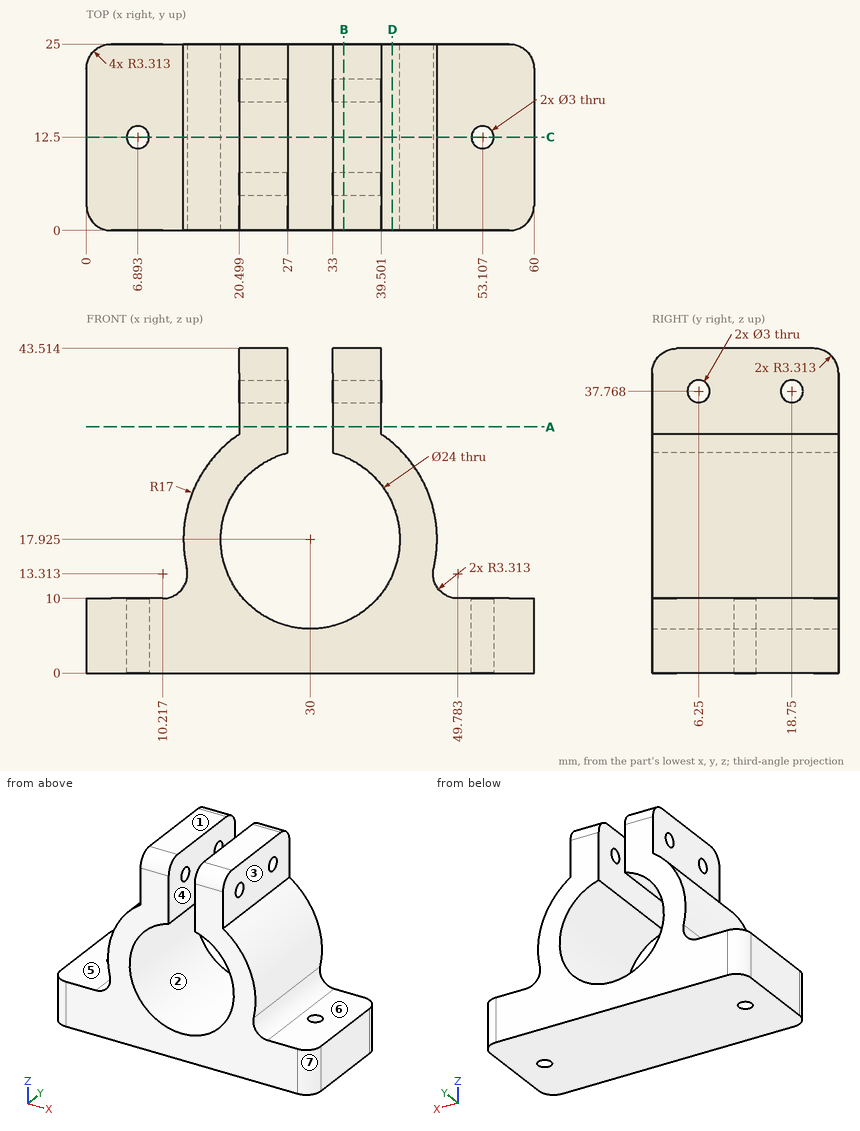
Input: dimensioned drawing with shaded views. Units: mm. Origin: part minimum x, y, z. A direction names the side the tool comes from. Round coordinates to 2 decimals unless told otherwise and drop trailing zeros. Write each loop counter-clockwise with the first axis right and the second up, starting at its lowest first coordinate (ties: lowest second). Pieces come first, ordered by that corner, then holes. Notation, with made-up numbers: (82, 52.5) -> (131, 52.5) arc R17 cw to (131, 83.5) -> close; hole circle Ø7 at (69.25, 12). An arc over 180 degrees is marked (long way). Use CSV: the item, a comma, the result in double quotes. Start each with the question number.
Q1. Reachability of the marked faces 4, 5, 6 and 7 from +Z, -Z, +X, -X, +Y, -Y: full face, straight path, thin tool, end or side. Return the list, or none.
Q2. Section B-B (x = 34.5). Return loops of the section in (y, z).
Q3. Section A-A (z = 33). Return loops of the section in (x, y).
Q4. Section C-C (y = 12.5). Return loops of the section in (x, z) (1 decimal), plus the area to 3 significant figures.
Q5. Pull-direction query (Z, two-part tool) for the marked faces 1, 2 and 3; classes: pulls with the +Z half, pulls with the -Z half, needs draft (parallel to the pull), parting line crosses it, or undercut.
Q6. Section D-D (x = 41). Return loops of the section in (y, z), plus the area to 3 significant figures.
Q7. First-contact query: pin 1 Ø4 at (y, z) = (12, 38) entering from -X; pin 2 Ø5 at (y, z) = (18.75, 37.77) entering from +X; pin 3 Ø3.5 at (x, y) = (53.11, 12.5) entering from +Z. Flat tips, straight axial feed; report the tip coordinate or a pass-through.
Q8. Line query: L1, parallel to X at y = 18.75, z = 34; L2, parallel to Z at x = 36.75, y = 18.75 (1 decimal); L3, parallel to Z at x = 24.5, y = 6.25 (1 decimal). Output: solid intervals per line, ascending.
Result sheet:
1,face 4,"+Z, +Y, -Y"
1,face 5,"+Z, -X, +Y, -Y"
1,face 6,"+Z, +X, +Y, -Y"
1,face 7,"+Z, -Z, +X, -Y"
2,outline,"(0, 0) -> (25, 0) -> (25, 6.8) -> (0, 6.8) -> close; (0, 29.05) -> (25, 29.05) -> (25, 40.2) arc R3.31 ccw to (21.69, 43.51) -> (3.31, 43.51) arc R3.31 ccw to (0, 40.2) -> close; hole circle Ø3 at (6.25, 37.77); hole circle Ø3 at (18.75, 37.77)"
3,outline,"(20.5, 0) -> (27, 0) -> (27, 25) -> (20.5, 25) -> close; (33, 0) -> (39.5, 0) -> (39.5, 25) -> (33, 25) -> close"
4,outline,"(0, 0) -> (5.4, 0) -> (5.4, 10) -> (0, 10) -> close; (8.4, 0) -> (51.6, 0) -> (51.6, 10) -> (49.8, 10) arc R3.3 cw to (46.6, 14.1) arc R17 ccw to (39.5, 32) -> (39.5, 43.5) -> (33, 43.5) -> (33, 29.5) arc R12 cw (long way) to (27, 29.5) -> (27, 43.5) -> (20.5, 43.5) -> (20.5, 32) arc R17 ccw to (13.4, 14.1) arc R3.3 cw to (10.2, 10) -> (8.4, 10) -> close; (54.6, 0) -> (60, 0) -> (60, 10) -> (54.6, 10) -> close"
4,area,"909 mm²"
5,face 1,"pulls with the +Z half"
5,face 2,"undercut"
5,face 3,"needs draft"
6,outline,"(0, 0) -> (25, 0) -> (25, 13.13) -> (0, 13.13) -> close; (0, 22.72) -> (25, 22.72) -> (25, 30.89) -> (0, 30.89) -> close"
6,area,"532 mm²"
7,pin 1,"x = 20.5"
7,pin 2,"x = 39.5"
7,pin 3,"z = 10"
8,L1,"20.5 to 27, 33 to 39.5"
8,L2,"0 to 8, 27.8 to 36.3, 39.3 to 43.5"
8,L3,"0 to 7.3, 28.6 to 36.3, 39.3 to 43.5"
